Input: dimensioned drawing with shaded views. Units: mm. Origin: part minimum x, y, z. Round coordinates to 2 decimals unless told otherwise and drop trailing zeros. Loops run counter-clockwise (first coordinate to the right, second up) from the corner with the lowest first, then second, coordinate; pieces in that order, holes last.
1) Section C-C, the plane x = 29.5. Return loops of the section in (y, z) (3 decimals), and give its area (3 significant figures).
2) Section B-B, the plane y = 36. Return loops of the section in (x, z) (3 decimals), and give its area (3 significant figures).
3) Section A-A, the plane z = 1.8. State how many separate pieces and enclosed holes the cut face has, and give its area (3 significant figures).
4) Ray query, line 1 along X through (y, z) = (57, 2.1) (3 decimals); line 2 along Y through (x, z) = (41.5, 1.7); line 3 along X through (y, z) = (20, 1.15) (3 decimals). Return the intervals inside material, ascending.
5) First-contact query: pin 1 (1.6 mm diameter, centred on y = 34, z = 1, fed in from -X) (3 decimals); pin 2 (1 mm diameter, centred on y = 58, z = 3, fed in from -X); pin 3 (1.6 mm diameter, centred on y = 40, z = 2.5, fed in from +X) (3 decimals). Flat tips, straight axial feed; report the tip coordinate or a pass-through.
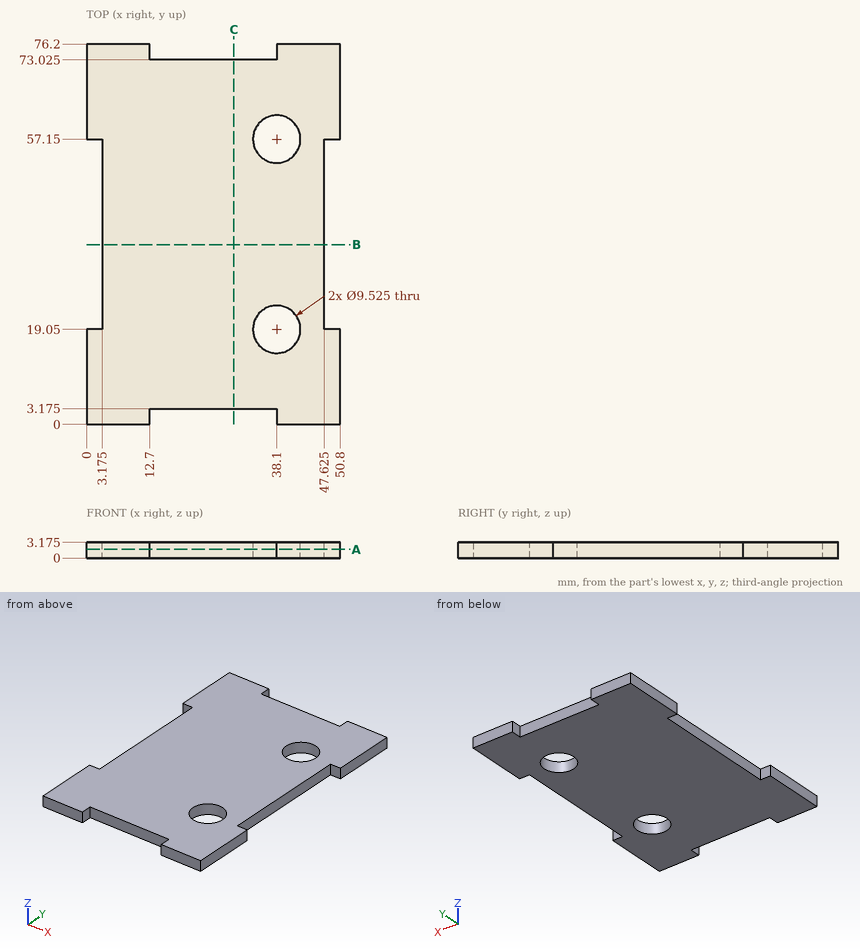
Final values:
1. outline: (3.175, 0) - (73.025, 0) - (73.025, 3.175) - (3.175, 3.175) - close
1. area: 222 mm2
2. outline: (3.175, 0) - (47.625, 0) - (47.625, 3.175) - (3.175, 3.175) - close
2. area: 141 mm2
3. separate pieces: 1
3. enclosed holes: 2
3. area: 3,330 mm2
4. line 1: x = 3.175 to 33.34, 42.86 to 47.625
4. line 2: y = 0 to 15.72, 22.38 to 53.82, 60.48 to 76.2
4. line 3: x = 3.175 to 33.433, 42.767 to 47.625
5. pin 1: stops at x = 3.175
5. pin 2: stops at x = 0
5. pin 3: stops at x = 47.625
